Source: CAD feature listing. Evaluate the final solid. Frame: model axes, mm. A direction names the side the tool comes from. Give positions to 0.01 mm unless a question says otherwise; leave off trailing zeros. Order: outer loops, then holes, each group sorted by start corner. A loop starts at its lowest first (then second) coordinate and runs counter-clockwise, first axis right, second up.
1) Section B-B, the plane z = 0. Return loops of the section in (x, y), plus the area to 3 significant figures.
2) Draft query along Z for faces 5 (the face through (24, -1, 0)), 6 (the face through (7, 4, 23)), 7 (the face through (18.479, 6.831, -17.793)). Return one class per face: released by +Z, released by -Z, zero draft, split by the parting line, or undercut.
3) First-contact query: P1, Ø6, axis at x = 19, z = -13.83, coming from the -Y side; P2, Ø4, axis at x = 17.5, z = -13, coming from the +Y side; P3, Ø2.5, axis at x = 7.5, y = -1, coming from the -Z side; P4, Ø1, axis at y = 1.5, z = -4, coming from the +X side. Flat tips, straight axial feed; report the tip coordinate or a pass-through.
4) Section C-C, the plane y = 5.25. Return loops of the section in (x, z), plus the area to 3 significant figures.
5) Material intervals for line 1 (Z direction, x = 6, y = 7.85); line 2 (Z direction, x = 15.5, y = 6.5); line 3 (X direction, y = 6, z = -15.5), sorted ascending.
6) Section D-D, the plane x = 40. Return loops of the section in (y, z), plus the area to 3 significant figures.
7) Access query for faces 1 (the face through (12, -1, -5)), 2 (the face through (12, -1, 5)), 3 (the face through (0, 4, 0)), 4 (the face through (5.48, 6.83, 8.84)). Directions: +Z, -Z, +X, -X, +Y, -Y. A direction counts if a zero-diameter tool reaches every point of the face in a straight line with its end or side. Return the directions, or none.
8) Section A-A, the plane x = 6. Return loops of the section in (y, z), plus the area to 3 significant figures.
```python
from build123d import *

# Parameters (mm, degrees)
EXTRUDE_1_DEPTH              = 9
SKETCH_2_W                   = 24
SKETCH_2_H                   = 10
EXTRUDE_2_DEPTH              = 3
HOLE_WIZARD_M4_1_D           = 4.5
HOLE_WIZARD_M4_1_DEPTH       = 9
HOLE_WIZARD_M4_1_CBORE_D     = 8
HOLE_WIZARD_M4_1_CBORE_DEPTH = 4.4
HOLE_WIZARD_M4_1_TIP         = 1.351936393
HOLE_WIZARD_M4_2_D           = 10
HOLE_WIZARD_M4_2_CBORE_D     = 13
HOLE_WIZARD_M4_2_CBORE_DEPTH = 3


with BuildPart() as part:
    # 스케치1 → 보스-돌출1 (new body)
    with BuildSketch(Plane(origin=(0, 0, 0), x_dir=(1, 0, 0), z_dir=(0, 1, 0))):
        with BuildLine():
            Line((0, 0), (0, 23))
            Line((0, 23), (13, 23))
            Line((13, 23), (44.075327331, 9.131905997))
            ThreePointArc((44.075327331, 9.131905997), (50, 0), (44.075327331, -9.131905997))
            Line((44.075327331, -9.131905997), (13, -23))
            Line((13, -23), (0, -23))
            Line((0, -23), (0, 0))
        make_face()
    extrude(amount=EXTRUDE_1_DEPTH)

    # 스케치2 → 보스-돌출2 (add)
    with BuildSketch(Plane.XZ):
        with Locations((12, 0)):
            Rectangle(SKETCH_2_W, SKETCH_2_H)
    extrude(amount=EXTRUDE_2_DEPTH)

    # M4 소켓 머리 캡 나사용 카운터보어1
    with Locations(Plane(origin=(0, 9, 0), x_dir=(1, 0, 0), z_dir=(0, 1, 0))):
        with Locations((6, 13.827116768), (19, 13.827116768), (6, -12.807083564), (19, -12.807083564)):
            CounterBoreHole(HOLE_WIZARD_M4_1_D / 2, HOLE_WIZARD_M4_1_CBORE_D / 2, HOLE_WIZARD_M4_1_CBORE_DEPTH, depth=HOLE_WIZARD_M4_1_DEPTH)
            with Locations((0, 0, -(HOLE_WIZARD_M4_1_DEPTH + HOLE_WIZARD_M4_1_TIP / 2))):  # 118° drill point
                Cone(0, HOLE_WIZARD_M4_1_D / 2, HOLE_WIZARD_M4_1_TIP, mode=Mode.SUBTRACT)

    # M4 소켓 머리 캡 나사용 카운터보어2 (through all)
    with Locations(Plane(origin=(0, 9, 0), x_dir=(1, 0, 0), z_dir=(0, 1, 0))):
        with Locations((40, 0)):
            CounterBoreHole(HOLE_WIZARD_M4_2_D / 2, HOLE_WIZARD_M4_2_CBORE_D / 2, HOLE_WIZARD_M4_2_CBORE_DEPTH)


solid = part.part
```
From the geometry:
1. outline: (0, -3) - (24, -3) - (24, 0) - (35, 0) - (35, 6) - (33.5, 6) - (33.5, 9) - (0, 9) - close; (45, 0) - (50, 0) - (50, 9) - (46.5, 9) - (46.5, 6) - (45, 6) - close
1. area: 423 mm2
2. face 5: zero draft
2. face 6: released by +Z
2. face 7: undercut
3. P1: stops at y = 0
3. P2: stops at y = 4.6
3. P3: stops at z = -23
3. P4: stops at x = 49.37
4. outline: (0, -23) - (13, -23) - (44.08, -9.13) arc R10 ccw to (44.08, 9.13) - (13, 23) - (0, 23) - close; hole circle Ø8 at (6, -13.83); hole circle Ø8 at (6, 12.81); hole circle Ø8 at (19, -13.83); hole circle Ø8 at (19, 12.81); hole circle Ø10 at (40, 0)
4. area: 1,390 mm2
5. line 1: z = -23 to -17.83, -9.83 to 8.81, 16.81 to 23
5. line 2: z = -21.88 to -15.76, -11.89 to 10.87, 14.74 to 21.88
5. line 3: x = 0 to 2.37, 9.63 to 15.37, 22.63 to 29.81
6. outline: (0, -10.95) - (9, -10.95) - (9, -6.5) - (6, -6.5) - (6, -5) - (0, -5) - close; (0, 5) - (6, 5) - (6, 6.5) - (9, 6.5) - (9, 10.95) - (0, 10.95) - close
6. area: 98.1 mm2
7. face 1: -Z, +X, -X, -Y
7. face 2: +Z, +X, -X, -Y
7. face 3: +Z, -Z, -X, +Y, -Y
7. face 4: +Y
8. outline: (-3, -5) - (0, -5) - (0, -11.58) - (4.6, -11.58) - (4.6, -9.83) - (9, -9.83) - (9, 8.81) - (4.6, 8.81) - (4.6, 10.56) - (0, 10.56) - (0, 5) - (-3, 5) - close; (0, -23) - (9, -23) - (9, -17.83) - (4.6, -17.83) - (4.6, -16.08) - (0, -16.08) - close; (0, 15.06) - (4.6, 15.06) - (4.6, 16.81) - (9, 16.81) - (9, 23) - (0, 23) - close
8. area: 332 mm2
